The drawing under review shows one solid part. Ordinate dimensions are in mm from its lowest x, y, z. Round coordinates to 2 decimals unless told otherwise and drop trailing zeros. Order: outer loops, then holes, each group sorted by start corner. A loop starts at its lowest first (then second) coordinate and runs counter-clockwise, first axis right, second up.
1) Mouldability with a two-part tool opening along Y and no side actions: class the marked faces 1, 2, 3 and 4 as pulls with the +Y half, pulls with the -Y half, needs draft (parallel to the pull), parting line crosses it, or undercut.
2) Clearance check with flat-ended pins moving along their axes: P1, Ø1.5, axis at x = 6, z = 2, coming from the +Y side; P2, Ø2, axis at x = 15, z = 2.5, coming from the +Y side. State where each tip first meets the part, or that it passes through.
3) To check wall thickness, follow L1, parallel to Y at x = 10, z = 2 (3 decimals); L2, parallel to X at y = 21.75, z = 5.5; L3, parallel to Y at x = 2, z = 0.5. State the ranges of each line that lie inside material, in increasing order.
4) Consider section B-B (x = 10). Give the boundary of the cut face in (y, z) (3 decimals).
5) Consider section D-D (y = 20.1). Give the boundary of the cut face in (x, z) (3 decimals).
6) Consider section C-C (z = 5). Give the boundary of the cut face in (x, y) (3 decimals).
7) Consider section A-A (y = 8). Give the boundary of the cut face in (x, z) (3 decimals), then the cut area to 4 significant figures.
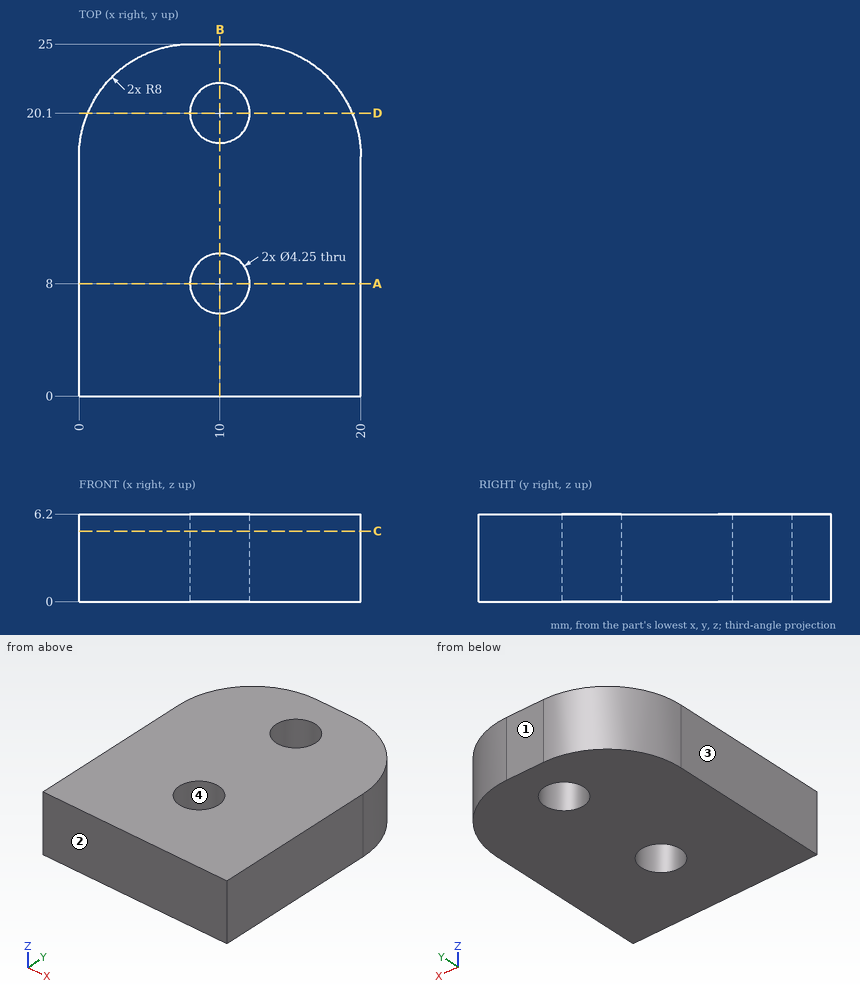
Answer below:
1. face 1: pulls with the +Y half
1. face 2: pulls with the -Y half
1. face 3: needs draft
1. face 4: undercut
2. P1: stops at y = 24.9
2. P2: stops at y = 24.75
3. L1: y = 0 to 5.875, 10.125 to 17.975, 22.225 to 25
3. L2: x = 1.56 to 8.66, 11.34 to 18.44
3. L3: y = 0 to 22.29
4. outline: (0, 0) - (5.875, 0) - (5.875, 6.2) - (0, 6.2) - close; (10.125, 0) - (17.975, 0) - (17.975, 6.2) - (10.125, 6.2) - close; (22.225, 0) - (25, 0) - (25, 6.2) - (22.225, 6.2) - close
5. outline: (0.625, 0) - (7.875, 0) - (7.875, 6.2) - (0.625, 6.2) - close; (12.125, 0) - (19.375, 0) - (19.375, 6.2) - (12.125, 6.2) - close
6. outline: (0, 0) - (20, 0) - (20, 17) arc R8 ccw to (12, 25) - (8, 25) arc R8 ccw to (0, 17) - close; hole circle Ø4.25 at (10, 8); hole circle Ø4.25 at (10, 20.1)
7. outline: (0, 0) - (7.875, 0) - (7.875, 6.2) - (0, 6.2) - close; (12.125, 0) - (20, 0) - (20, 6.2) - (12.125, 6.2) - close
7. area: 97.65 mm2
